Geometry: see drawing. Coordinates: mm, zero at the bounding-box minimum. A direction names the side the tool comes from. Round coordinates to 2 decimals unless told otherwise and drop trailing zeros. Loops run counter-clockwise (first coordinate to the right, second up) from the corner with the lowest first, then second, coordinate; pieces in that order, holes last. Notation, with made-up numbers: (55, 1.25) - (94, 1.25) arc R21 cw to (94, 23.25) - close; hole circle Ø11 at (44, 3.5). An arc over 180 degrees is marked (long way). One line per question, with ' | ' between items. Start each with the question number.
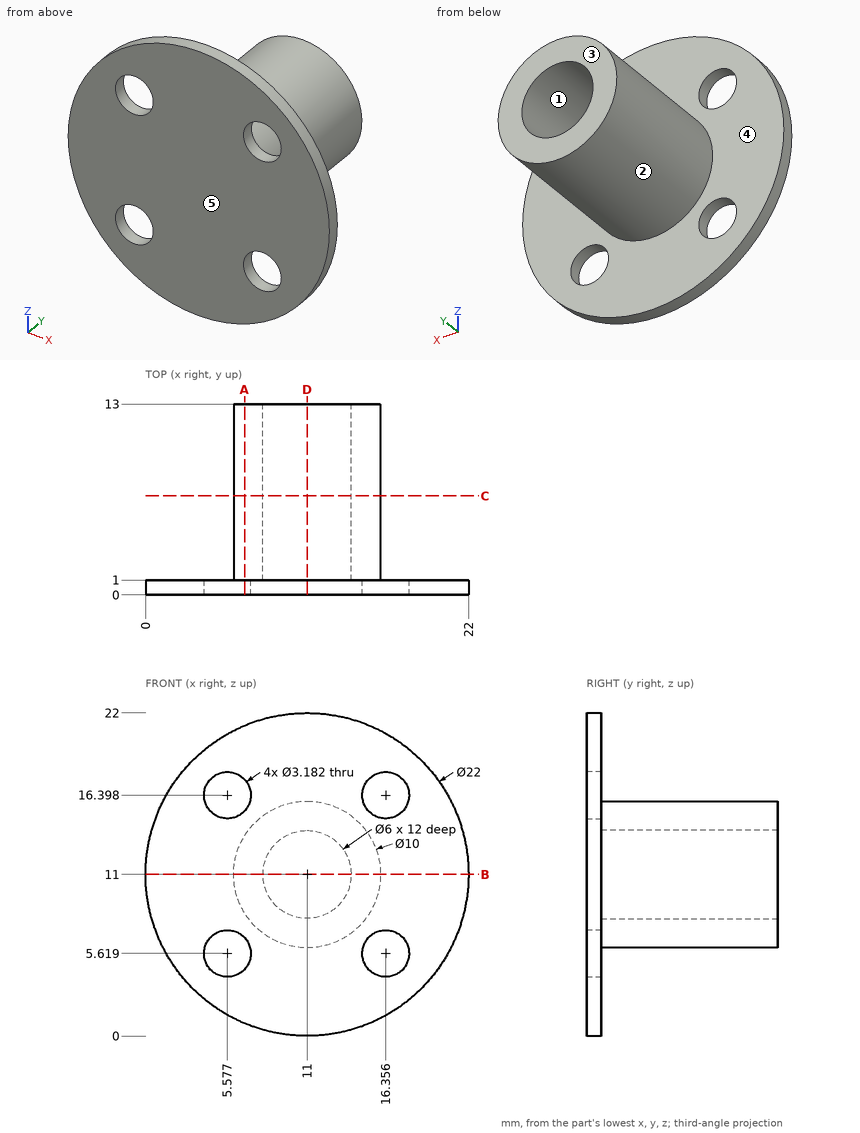
(1) Pull-direction query (X, two-part tool) for the marked faces 1, 2 and 3; classes: released by +X, released by -X, zero draft, split by the parting line, or undercut.
(2) Section C-C, the plane y = 6.75. Output: boundary loops of the cut face in (x, z).
(3) Reachability of the marked faces 4 and 5 from +Z, -Z, +X, -X, +Y, -Y: full face, straight path, thin tool, end or side. Return the list, or none.
(4) Line query: line 1 along X through (y, z) = (9, 7); line 2 along X through (y, z) = (5, 11); line 3 along Y through (x, z) = (10.75, 11). Output: solid intervals per line, ascending. Write a range as from..to.
(5) Section A-A, the plane x = 6.75. Output: boundary loops of the cut face in (y, z), plus the area to 3 significant figures.
(6) Section D-D, the plane x = 11. Output: boundary loops of the cut face in (y, z).
(7) Section B-B, the plane z = 11. Output: boundary loops of the cut face in (x, y).
(8) Pin query (flat end, axial travel): P1, Ø3.5, axis at x = 16.36, z = 5.62, coming from the +Y side; P2, Ø4, axis at y = 7.5, z = 13, coming from the -X side; P3, Ø5.5, axis at x = 11, z = 11, coming from the -Y side; P4, Ø1, axis at x = 13, y = 4.5, coming from the +Z side. Return the tip coordinate at first contact, or that it passes through.
Derived:
1) face 1: undercut | face 2: split by the parting line | face 3: zero draft
2) outline: circle Ø10 at (11, 11); hole circle Ø6 at (11, 11)
3) face 4: +Y | face 5: +Z, -Z, +X, -X, -Y
4) line 1: x = 8..14 | line 2: x = 6..8, 14..16 | line 3: y = 0..1
5) outline: (0, 0.85) - (1, 0.85) - (1, 4.54) - (0, 4.54) - close; (0, 6.69) - (1, 6.69) - (1, 8.37) - (13, 8.37) - (13, 13.63) - (1, 13.63) - (1, 15.32) - (0, 15.32) - close; (0, 17.47) - (1, 17.47) - (1, 21.15) - (0, 21.15) - close | area: 79.2 mm²
6) outline: (0, 0) - (1, 0) - (1, 6) - (13, 6) - (13, 8) - (1, 8) - (1, 14) - (13, 14) - (13, 16) - (1, 16) - (1, 22) - (0, 22) - close
7) outline: (0, 0) - (22, 0) - (22, 1) - (16, 1) - (16, 13) - (14, 13) - (14, 1) - (8, 1) - (8, 13) - (6, 13) - (6, 1) - (0, 1) - close
8) P1: stops at y = 1 | P2: stops at x = 6 | P3: stops at y = 0 | P4: stops at z = 15.77
